from build123d import *

# Parameters (mm, degrees)
BOSS_EXTRUDE1_DEPTH                            = 8.5
CBORE_FOR_M2_SOCKET_HEAD_CAP_SCREW1_AT_2_COUNT = 2
CBORE_FOR_M2_SOCKET_HEAD_CAP_SCREW1_AT_2_PITCH = 61
SKETCH8_W                                      = 53
SKETCH8_H                                      = 1
CUT_EXTRUDE1_DEPTH                             = 9.5
M2X0_4_TAPPED_HOLE8_D                          = 1.6
SKETCH14_W                                     = 83
SKETCH14_H                                     = 1.6
CUT_EXTRUDE2_DEPTH                             = 10
M2X0_4_TAPPED_HOLE7_D                          = 1.6
M2X0_4_TAPPED_HOLE6_D                          = 1.6
M2X0_4_TAPPED_HOLE6_DEPTH                      = 5.2
M2X0_4_TAPPED_HOLE6_TIP                        = 0.480688495


with BuildPart() as part:
    # Sketch1 → Boss-Extrude1 (new body)
    with BuildSketch(Plane.XY):
        Polygon((53, -3), (68, -3), (68, -6), (-15, -6), (-15, -3), (0, -3), (0, 0), (53, 0), align=None)
    extrude(amount=BOSS_EXTRUDE1_DEPTH)

    # Sketch4 → CBORE for M2 Socket Head Cap Screw1 (revolve, cut)
    with BuildSketch(Plane(origin=(-4, -6, 2.75), x_dir=(0, 0, -1), z_dir=(1, 0, 0))):
        Polygon((0, 0), (0, 6), (1.2, 6), (1.2, 2.025), (1.225, 2), (2.2, 2), (2.2, 0), align=None)
    cbore_for_m2_socket_head_cap_screw1 = revolve(axis=Axis((-4, -12.35, 2.75), (0, 1, 0)), mode=Mode.SUBTRACT)

    # CBORE for M2 Socket Head Cap Screw1 at 2: CBORE for M2 Socket Head Cap Screw1 ×2
    with Locations(*[(i * CBORE_FOR_M2_SOCKET_HEAD_CAP_SCREW1_AT_2_PITCH, 0, 0) for i in range(1, CBORE_FOR_M2_SOCKET_HEAD_CAP_SCREW1_AT_2_COUNT)]):
        add(cbore_for_m2_socket_head_cap_screw1, mode=Mode.SUBTRACT)

    # Sketch8 → Cut-Extrude1 (cut, through all)
    with BuildSketch(Plane.XY.offset(8.5)):
        with Locations((26.5, -0.5)):
            Rectangle(SKETCH8_W, SKETCH8_H)
    extrude(amount=-CUT_EXTRUDE1_DEPTH, mode=Mode.SUBTRACT)

    # M2x0.4 Tapped Hole8 (through all)
    with Locations(Plane.XY.offset(8.5)):
        with Locations((2, -4.5), (51, -4.5)):
            Hole(M2X0_4_TAPPED_HOLE8_D / 2)

    # Sketch14 → Cut-Extrude2 (cut)
    with BuildSketch(Plane.XZ.offset(6)):
        with Locations((26.5, 7.7)):
            Rectangle(SKETCH14_W, SKETCH14_H)
    extrude(amount=-CUT_EXTRUDE2_DEPTH, mode=Mode.SUBTRACT)

    # M2x0.4 Tapped Hole7 (through all)
    with Locations(Plane(origin=(0, -6, 0), x_dir=(-1, 0, 0), z_dir=(0, -1, 0))):
        with Locations((8, -4.2), (-61, -4.2)):
            Hole(M2X0_4_TAPPED_HOLE7_D / 2)

    # M2x0.4 Tapped Hole6
    with Locations(Plane(origin=(0, -6, 0), x_dir=(-1, 0, 0), z_dir=(0, -1, 0))):
        with Locations((-26.5, -4)):
            Hole(M2X0_4_TAPPED_HOLE6_D / 2, depth=M2X0_4_TAPPED_HOLE6_DEPTH)
            with Locations((0, 0, -(M2X0_4_TAPPED_HOLE6_DEPTH + M2X0_4_TAPPED_HOLE6_TIP / 2))):  # 118° drill point
                Cone(0, M2X0_4_TAPPED_HOLE6_D / 2, M2X0_4_TAPPED_HOLE6_TIP, mode=Mode.SUBTRACT)


solid = part.part
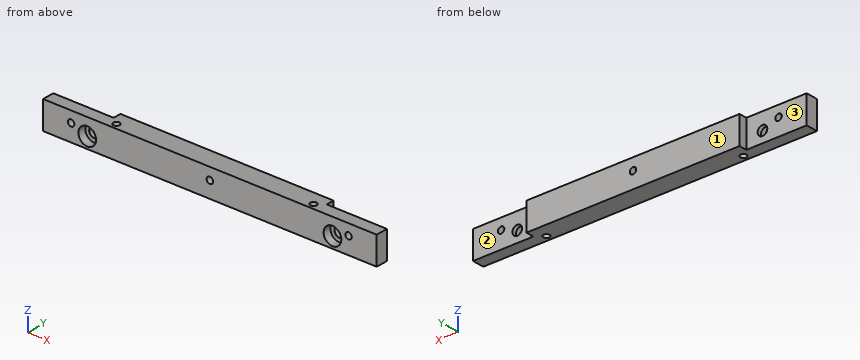
Design review of the part built by this model. Coordinates are the model's own, in mm. Face numbers are marked on the shaded views. A direction names the side the tool comes from. Round coordinates to 2 decimals unless told otherwise and drop trailing zeros. Write each loop counter-clockwise with the first axis right and the second up, starting at its lowest first coordinate (ties: lowest second). Pieces come first, ordered by that corner, then holes. Notation, with made-up numbers: (73, 64) - (87, 64) arc R19 ccw to (87, 88) - close; hole circle Ø6 at (22.5, 48). An arc over 180 degrees is marked (long way). Return JSON: item names as keys, results as strings. Group by question number.
Item 1: We need section A-A on x = -4. Write out the cut boundary in (y, z) (3 decimals), and give its area (3 significant figures).
Item 2: For probe 1 along X at (y, z) = (-3.2, 2.75); probe 2 along X at (y, z) = (-4.65, 6.5); probe 3 along X at (y, z) = (-4.65, 2.75), list the stretches that pass through material, from the lowest coordinate up. Write a range as [from, to].
Item 3: We need section B-B on z = 6. Write out the cut boundary in (x, y), and give its area (3 significant figures).
Item 4: We need section D-D on x = 51. Write out the cut boundary in (y, z), and give its area (3 significant figures).
Item 5: Insertion check: P1, Ø1.4, axis at x = 26.5, z = 4, coming from the +Y side; P2, Ø4, axis at x = -4, z = 2.75, coming from the +Y side; P3, Ø4, axis at x = -4, z = 2.75, coming from the -Y side; P4, Ø1, axis at y = -2, z = 2, coming from the +X side. Each pin has a flat end and moves straight along its axis. Give the tip position at first contact, or say it passes through.
Item 6: We need section C-C on x = 61. Write out the cut boundary in (y, z), and give its area (3 significant figures).
Item 7: Machinability: for the marked faces 1, 2 and 3, which of the approach directions +Z, -Z, +X, -X, +Y, -Y give a long, thin tool a straight path to every point of the face, cutting with its end or side? Answer none if there is none.
Model answer:
{
 "1": {"outline": "(-6, 0) - (-3, 0) - (-3, 1.55) - (-3.975, 1.55) - (-4, 1.525) - (-4, 0.55) - (-6, 0.55) - close; (-6, 4.95) - (-4, 4.95) - (-4, 3.975) - (-3.975, 3.95) - (-3, 3.95) - (-3, 6.9) - (-6, 6.9) - close", "area": "9.50 mm²"},
 "2": {"probe 1": "x = [-15, -5.2], [-2.8, 55.8], [58.2, 68]", "probe 2": "x = [-15, 1.21], [2.79, 50.21], [51.79, 68]", "probe 3": "x = [-15, -6.2], [-1.8, 1.21], [2.79, 50.21], [51.79, 54.8], [59.2, 68]"},
 "3": {"outline": "(-15, -6) - (68, -6) - (68, -3) - (53, -3) - (53, -1) - (0, -1) - (0, -3) - (-15, -3) - close; hole circle Ø1.6 at (2, -4.5); hole circle Ø1.6 at (51, -4.5)", "area": "351 mm²"},
 "4": {"outline": "(-6, 0) - (-5.3, 0) - (-5.3, 6.9) - (-6, 6.9) - close; (-3.7, 0) - (-1, 0) - (-1, 6.9) - (-3.7, 6.9) - close", "area": "23.5 mm²"},
 "5": {"P1": "passes through", "P2": "stops at y = -3", "P3": "stops at y = -4", "P4": "stops at x = 53"},
 "6": {"outline": "(-6, 0) - (-3, 0) - (-3, 3.4) - (-6, 3.4) - close; (-6, 5) - (-3, 5) - (-3, 6.9) - (-6, 6.9) - close", "area": "15.9 mm²"},
 "7": {"face 1": "+Z, -Z, +X, -X, +Y", "face 2": "+Z, -Z, +X, +Y", "face 3": "+Z, -Z, -X, +Y"}
}
